```python
from build123d import *

# Parameters (mm, degrees)
BOSS_EXTRUDE1_DEPTH     = 1
SKETCH3_W               = 56
SKETCH3_H               = 146
CUT_EXTRUDE2_DEPTH      = 10
CUT_EXTRUDE4_DEPTH      = 607.465859368
CUT_EXTRUDE4_DEPTH_BACK = 607.465859368
SKETCH4_W               = 323.526326174
SKETCH4_H               = 73.784869865
SKETCH5_W               = 0.9
SKETCH5_H               = 318.91
BOSS_EXTRUDE2_DEPTH     = 1
CUT_EXTRUDE6_DEPTH      = 558.674774622
CUT_EXTRUDE6_DEPTH_BACK = 11.5
SKETCH6_W               = 184.6
SKETCH6_H               = 110.039837523
CUT_EXTRUDE7_DEPTH      = 558.674774622
CUT_EXTRUDE7_DEPTH_BACK = 558.674774622
SKETCH7_W               = 27
SKETCH7_H               = 48.713018504
CUT_EXTRUDE8_DEPTH      = 558.674774622
CUT_EXTRUDE8_DEPTH_BACK = 558.674774622
SKETCH8_W               = 268.184865131
SKETCH8_H               = 40.991987157
BOSS_EXTRUDE3_DEPTH     = 1
CUT_EXTRUDE9_DEPTH      = 559.688754003
CUT_EXTRUDE9_DEPTH_BACK = 559.688754003


with BuildPart() as part:
    # Sketch1 → Boss-Extrude1 (new body)
    with BuildSketch(Plane(origin=(0, 0, 0), x_dir=(1, 0, 0), z_dir=(0, 1, 0))):
        Polygon((-292.25, 307.91829646), (-292.25, -10.99170354), (292.25, -10.99170354), (292.25, 307.91829646), (0, 531.403590578), align=None)
    extrude(amount=BOSS_EXTRUDE1_DEPTH)

    # Sketch3 → Cut-Extrude2 (cut)
    with BuildSketch(Plane(origin=(0, 1, 0), x_dir=(1, 0, 0), z_dir=(0, 1, 0))):
        with Locations((-204.688244909, 164.834464834)):
            Rectangle(SKETCH3_W, SKETCH3_H)
        with Locations((205.588244909, 164.834464834)):
            Rectangle(SKETCH3_W, SKETCH3_H)
    extrude(amount=-CUT_EXTRUDE2_DEPTH, mode=Mode.SUBTRACT)

    # Sketch4 → Cut-Extrude4 (cut, two sides: drawn at the far end of the back side and taken through both)
    with BuildSketch(Plane(origin=(0, 1, 0), x_dir=(1, 0, 0), z_dir=(0, 1, 0)).offset(-CUT_EXTRUDE4_DEPTH_BACK)):
        with Locations((-21.051035773, 511.300731392)):
            Rectangle(SKETCH4_W, SKETCH4_H)
    extrude(amount=CUT_EXTRUDE4_DEPTH + CUT_EXTRUDE4_DEPTH_BACK, mode=Mode.SUBTRACT)

    # Sketch5 → Boss-Extrude2 (add)
    with BuildSketch(Plane(origin=(0, 1, 0), x_dir=(1, 0, 0), z_dir=(0, 1, 0))):
        with Locations((292.7, 148.46329646)):
            Rectangle(SKETCH5_W, SKETCH5_H)
    extrude(amount=-BOSS_EXTRUDE2_DEPTH)

    # Sketch6 → Cut-Extrude6 (cut, two sides: drawn at the far end of the back side and taken through both)
    with BuildSketch(Plane(origin=(0, 1, 0), x_dir=(1, 0, 0), z_dir=(0, 1, 0)).offset(-CUT_EXTRUDE6_DEPTH_BACK)):
        with Locations((-4.55, 399.428215222)):
            Rectangle(SKETCH6_W, SKETCH6_H)
    extrude(amount=CUT_EXTRUDE6_DEPTH + CUT_EXTRUDE6_DEPTH_BACK, mode=Mode.SUBTRACT)

    # Sketch7 → Cut-Extrude7 (cut, two sides: drawn at the far end of the back side and taken through both)
    with BuildSketch(Plane(origin=(0, 1, 0), x_dir=(1, 0, 0), z_dir=(0, 1, 0)).offset(-CUT_EXTRUDE7_DEPTH_BACK)):
        with Locations((-146.945577185, 378.369305764)):
            Rectangle(SKETCH7_W, SKETCH7_H)
        with Locations((146.945577185, 378.369305764)):
            Rectangle(SKETCH7_W, SKETCH7_H)
    extrude(amount=CUT_EXTRUDE7_DEPTH + CUT_EXTRUDE7_DEPTH_BACK, mode=Mode.SUBTRACT)

    # Sketch8 → Cut-Extrude8 (cut, two sides: drawn at the far end of the back side and taken through both)
    with BuildSketch(Plane(origin=(0, 1, 0), x_dir=(1, 0, 0), z_dir=(0, 1, 0)).offset(-CUT_EXTRUDE8_DEPTH_BACK)):
        with Locations((19.664678058, 474.092644014)):
            Rectangle(SKETCH8_W, SKETCH8_H)
    extrude(amount=CUT_EXTRUDE8_DEPTH + CUT_EXTRUDE8_DEPTH_BACK, mode=Mode.SUBTRACT)

    # Sketch9 → Boss-Extrude3 (add)
    with BuildSketch(Plane(origin=(0, 1, 0), x_dir=(1, 0, 0), z_dir=(0, 1, 0))):
        Polygon((-292.25, 307.91829646), (-291.361, 343.51929646), (-114.760549692, 475.59983321), (-97.590157883, 473.756060592), (-96.85, 453.596650435), (-101.74753711, 453.596650435), align=None)
        Polygon((87.75, 453.596650435), (87.75, 474.677946901), (122.261, 473.51929646), (293.15, 344.40829646), (292.25, 307.91829646), (101.74753711, 453.596650435), align=None)
    extrude(amount=-BOSS_EXTRUDE3_DEPTH)

    # Sketch10 → Cut-Extrude9 (cut, two sides: drawn at the far end of the back side and taken through both)
    with BuildSketch(Plane(origin=(0, 1, 0), x_dir=(1, 0, 0), z_dir=(0, 1, 0)).offset(-CUT_EXTRUDE9_DEPTH_BACK)):
        Polygon((87.75, 474.677946901), (98.639, 474.40829646), (98.639, 343.51929646), (87.75, 343.51929646), align=None)
    extrude(amount=CUT_EXTRUDE9_DEPTH + CUT_EXTRUDE9_DEPTH_BACK, mode=Mode.SUBTRACT)


solid = part.part
```
Geometry: final body of the model. Coordinates: model frame, mm. Round coordinates to 2 decimals unless told otherwise and drop trailing zeros. Loops run counter-clockwise (first coordinate to the right, second up) from the corner with the lowest first, then second, coordinate; pieces in that order, holes last. Notation, with made-up numbers: (75, 84.5) -> (132, 84.5) arc R15 cw to (132, 102.5) -> close; hole circle Ø8 at (80, 86.25). An arc over 180 degrees is marked (long way). Use one line per item in the form item = value. Start each with the question number.
1) First-contact query: P1, Ø0.5, axis at x = -148, y = 0.5, coming from the -Z side; P2, Ø0.5, axis at x = 202.5, y = 0.5, coming from the -Z side. Flat tips, straight axial feed; report the tip coordinate or a pass-through.
2) Line query: L1, parallel to X at y = 0.85, z = -134.5; L2, parallel to X at y = 0.1, z = -356.5; L3, parallel to X at y = 0.4, z = -357. Output: solid intervals per line, ascending.
3) Section D-D on z = -209. Output: boundary loops of the cut face in (x, y).
4) Section A-A on z = -442.5. Output: boundary loops of the cut face in (x, y), then the cut area to 3 significant figures.
5) Section B-B on y = 0.55. Give the number of separate pieces and of enclosed holes in the cut face, then the cut area to 3 significant figures.
6) Section C-C on x = -187.5. Output: boundary loops of the cut face in (y, z), then the cut area to 3 significant figures.
Response:
q1.P1 = -450.93
q1.P2 = -413.09
q2.L1 = -292.25 to -232.69, -176.69 to 177.59, 233.59 to 293.15
q2.L2 = -274 to -160.45, -133.45 to -96.85, 98.64 to 133.45, 160.45 to 277.15
q2.L3 = -273.34 to -160.45, -133.45 to -96.85, 98.64 to 133.45, 160.45 to 276.48
q3.outline = (-292.25, 0) -> (-232.69, 0) -> (-232.69, 1) -> (-292.25, 1) -> close; (-176.69, 0) -> (177.59, 0) -> (177.59, 1) -> (-176.69, 1) -> close; (233.59, 0) -> (293.15, 0) -> (293.15, 1) -> (233.59, 1) -> close
q4.outline = (-159.02, 0) -> (-96.85, 0) -> (-96.85, 1) -> (-159.02, 1) -> close; (98.64, 0) -> (163.32, 0) -> (163.32, 1) -> (98.64, 1) -> close
q4.area = 127 mm^2
q5.separate_pieces = 1
q5.enclosed_holes = 4
q5.area = 217,000 mm^2
q6.outline = (0, -421.2) -> (1, -421.2) -> (1, -237.83) -> (0, -237.83) -> close; (0, -91.83) -> (1, -91.83) -> (1, 10.99) -> (0, 10.99) -> close
q6.area = 286 mm^2
